Read the model definition and answer for the solid it produces. Units are mm, in the model's axes. Face numbers are marked on the shaded views. A direction names the side the tool comes from. Coordinates: 2 decimals unless noted, no trailing zeros. Write each loop counter-clockwise with the first axis right and the second up, starting at its lowest first coordinate (ties: lowest second). Pieces come first, ordered by that corner, then holes. Notation, with made-up numbers: (14.5, 31) -> (54.5, 31) arc R26 cw to (54.5, 64) -> close; hole circle Ø5 at (12.25, 84). An arc over 180 degrees is marked (long way). One line per item, written item: value. Start each with the question number.
from build123d import *


with BuildPart() as part:
    # Sketch1 → Revolve7 (revolve)
    with BuildSketch(Plane.XY, mode=Mode.PRIVATE) as revolve7_sk:
        with BuildLine():
            Line((10.276772921, 1.166214565), (13.032359095, 2.0955))
            Line((13.032359095, 2.0955), (13.032359095, 0))
            Line((13.032359095, 0), (13.462, 0))
            Line((13.462, 0), (13.462, 1.8415))
            ThreePointArc((13.462, 1.8415), (13.536394878, 2.021105122), (13.716, 2.0955))
            Line((13.716, 2.0955), (25.1714, 2.0955))
            Line((25.1714, 2.0955), (25.1714, 3.3655))
            Line((25.1714, 3.3655), (27.178, 4.8895))
            ThreePointArc((27.178, 4.8895), (27.914506706, 5.666579226), (28.2194, 6.6929))
            Line((28.2194, 6.6929), (1.27, 6.6929))
            Line((1.27, 6.6929), (0.155422631, 6.6929))
            Line((0.155422631, 6.6929), (0.155422631, 6.662703245))
            ThreePointArc((0.155422631, 6.662703245), (0.183846403, 6.474846172), (0.266573119, 6.303806757))
            Line((0.266573119, 6.303806757), (0.906722652, 5.36943701))
            ThreePointArc((0.906722652, 5.36943701), (1.160671231, 4.899340794), (1.310662302, 4.386522101))
            ThreePointArc((1.310662302, 4.386522101), (1.666264155, 3.476843471), (2.338850191, 2.768609109))
            ThreePointArc((2.338850191, 2.768609109), (5.95509585, 1.158024647), (9.912867233, 1.072815189))
            ThreePointArc((9.912867233, 1.072815189), (10.096549324, 1.112777329), (10.276772921, 1.166214565))
        make_face()
    revolve(revolve7_sk.sketch.rotate(Axis((0, 6.6929, 0), (1, 0, 0)), 270), axis=Axis((0, 6.6929, 0), (1, 0, 0)))


solid = part.part
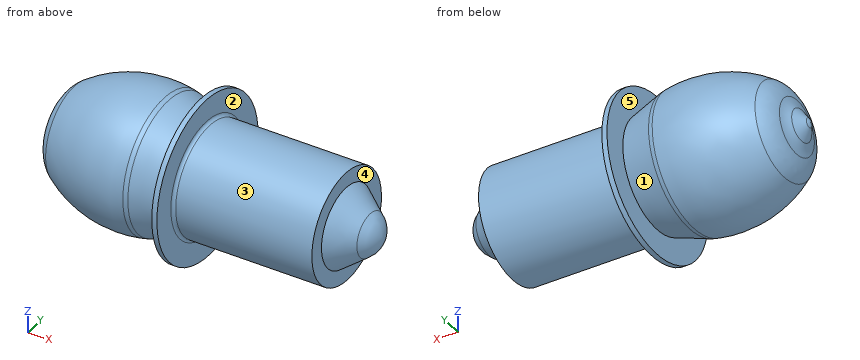
1. For a pull along X with two mould halves and no side action, classify the marked faces 3, 4 and 5 as +X half, -X half, draft (parallel to the pull), parting line (faces both ways), or undercut.
2. A cutting plane is placed at A-A on x = 24.5. Give the vertices of the cut face in (y, z), then the cut area to 3 significant figures.
3. Find the intervals of material crossed by probe 1 along Z at (x, y) = (4.5, 9.75); probe 2 along Y at (x, z) = (3.5, -2); probe 3 along Y at (x, z) = (4.5, -0.75), in increasing order. Write a range as from..to.
4. Given pin 1 (5 mm diameter, centred on x = 9.5, y = 12, fed in from +Z); pin 2 (8 mm diameter, centred on x = 22.5, z = -3, fed in from -Y); pin 3 (8 mm diameter, centred on x = 7.5, z = 4, fed in from -Y), each flat-ended and moving along its own axis, determine where each tip first touches the part or whether it passes through.
5. A tool of negligible diameter and unlimited length cuts with its end or side. For the marked faces 1 and 2, from which of +Z, -Z, +X, -X, +Y, -Y can it reach the whole face along a straight path? Write none if from no direction.
Derived:
1. face 3: draft
1. face 4: +X half
1. face 5: undercut
2. outline: circle Ø9.19 at (6.69, 0)
2. area: 66.4 mm2
3. probe 1: z = -4.07..4.07
3. probe 2: y = 2.51..10.88
3. probe 3: y = 1.66..11.73
4. pin 1: stops at z = 4.98
4. pin 2: stops at y = 2.1
4. pin 3: stops at y = 0.92
5. face 1: none
5. face 2: +X
